For this review, take the finished solid that the model builds, in its own axes (mm). A direction names the side the tool comes from. Coordinates: 2 decimals unless noted, no trailing zeros. Write each loop counter-clockwise with the first axis right and the second up, starting at its lowest first coordinate (ties: lowest second). Pieces come first, ordered by that corner, then holes. Notation, with made-up numbers: (54, 52.5) -> (103, 52.5) arc R16 ccw to (103, 67.5) -> close; hole circle Ø1 at (-19, -2.5). An arc over 180 degrees is marked (long way). Put each result on its own line as item: value. Start each with the question number.
Item 1: Consider section D-D on z = 3. Give the boundary of the cut face in (x, y).
Item 2: Consider section C-C on x = 68.5. Give the boundary of the cut face in (y, z).
Item 3: For faces 4 (the flat face through (137.496, -8.802, 8.208)), 5 (the cylindrical face through (134.365, 3.488, -8.837)), 6 (the flat face through (134.92, 11, -4)), list the 3-axis set-ups (+Z, -Z, +X, -X, +Y, -Y) from which the entire face can be reached by the end or side of a thin tool; tool diameter is ignored.
Item 4: Consider section A-A on y = 0. Give the boundary of the cut face in (x, z).
Item 5: The part is to be moulded in two halves that separate along X. For faces 1 (the flat face through (0, 0, 0)), 2 (the flat face through (137, 12, 0)), 3 (the flat face through (134.92, -11, 4)), say which applies: +X half, -X half, draft (parallel to the pull), parting line (faces both ways), or undercut.
Item 6: To check wall thickness, follow L1, parallel to X at y = -0.5, z = -10; L2, parallel to X at y = 18, z = -11.5; L3, parallel to Y at x = 121.5, z = -14.5. State the ranges of each line that lie inside material, in increasing order.
Item 7: Insertion check: P1, Ø12, axis at x = 123, z = 0.5, coming from the +Y side; P2, Ø4, axis at x = 75.5, z = -7, coming from the -Y side; P3, Ø8, axis at y = 14.5, z = 18, coming from the +X side. Each pin has a flat end and moves straight along its axis. Give the tip position at first contact, or say it passes through.
Item 8: Consider section B-B on z = -3.5. Give the boundary of the cut face in (x, y), and give its area (3 significant figures).
Autodesk Inventor part; units mm, degrees
ref_plane "YZ Plane" through (0, 0, 0) normal (1, 0, 0) x (0, 1, 0)
ref_plane "XZ Plane" through (0, 0, 0) normal (0, 1, 0) x (-1, 0, 0)
ref_plane "XY Plane" through (0, 0, 0) normal (0, 0, 1) x (1, 0, 0)
sketch "Sketch1" plane through (0, 0, 0) normal (1, 0, 0) x (0, 1, 0)
  circle A0 centre (0, 0) radius 15
  dimension "d0" = 30
extrude "Extrusion1" add sketch "Sketch1" along normal blind 140
sketch "Sketch2" plane through (140, 0, 0) normal (1, 0, 0) x (0, 0, -1)
  circle A0 centre (0, 0) radius 9.5
  circle A1 centre (0, 0) radius 15
  line L0 (0, 15) -> (0, 9.5)
  line L1 (0, -9.5) -> (0, -15)
  line L2 (10.23, 10.9703) -> (6.479, 6.9479)
  line L3 (-10.23, -10.9703) -> (-6.479, -6.9479)
  dimension "d3" = 19
  dimension "d4" = 43
  dimension "d5" = 43
extrude "Extrusion2" cut sketch "Sketch2" against normal blind 11.43 contours A0 L2 A1 L1 | A0 L3 A1 L0
sketch "Sketch3" plane through (128.57, 0, 0) normal (1, 0, 0) x (0, 0, -1)
  circle A0 centre (0, 0) radius 15
  circle A1 centre (0, 0) radius 9.5
  dimension "d22" = 19
  dimension "d23" = 30
extrude "Extrusion3" cut sketch "Sketch3" along normal blind 6.35
sketch "Sketch6" plane through (0, 0, 0) normal (-1, 0, 0) x (0, 0, 1)
  circle A0 centre (0, 0) radius 22.5
  dimension "d16" = 45
extrude "Extrusion6" add sketch "Sketch6" against normal up to surface (128.57 mm away)
sketch "Sketch7" plane through (0, 0, 0) normal (-1, 0, 0) x (0, 0, 1)
  circle A0 centre (0, 0) radius 15
  circle A1 centre (0, 0) radius 22.5
  dimension "d19" = 30
extrude "Extrusion7" cut sketch "Sketch7" against normal blind 11.43
sketch "Sketch8" plane through (140, 0, 0) normal (1, 0, 0) x (0, 0, -1)
  arc A0 (10.23, 10.9703) -> (0, 15) centre (0, 0) ccw
  circle A1 centre (0, 0) radius 15
  circle A2 centre (0, 0) radius 14.5
  point P0 (0, 15)
  dimension "d24" = 0.5
extrude "Extrusion8" cut sketch "Sketch8" against normal up to surface (5.08 mm away)
properties part number "spool axle" material "PLA"
Return value:
1. outline: (0, -14.7) -> (11.43, -14.7) -> (11.43, -22.3) -> (128.57, -22.3) -> (128.57, -9.01) -> (134.92, -9.01) -> (134.92, -14.19) -> (140, -14.19) -> (140, 9.01) -> (128.57, 9.01) -> (128.57, 22.3) -> (11.43, 22.3) -> (11.43, 14.7) -> (0, 14.7) -> close
2. outline: circle Ø45 at (0, 0)
3. face 4: +Z, +X
3. face 5: none
3. face 6: -Z, +Y
4. outline: (0, -15) -> (11.43, -15) -> (11.43, -22.5) -> (128.57, -22.5) -> (128.57, -9.5) -> (140, -9.5) -> (140, 9.5) -> (128.57, 9.5) -> (128.57, 22.5) -> (11.43, 22.5) -> (11.43, 15) -> (0, 15) -> close
5. face 1: -X half
5. face 2: draft
5. face 3: undercut
6. L1: 0 to 128.57
6. L2: 11.43 to 128.57
6. L3: -17.2 to 17.2
7. P1: y = 22.5
7. P2: y = -21.94
7. P3: x = 128.57
8. outline: (0, -14.59) -> (11.43, -14.59) -> (11.43, -22.23) -> (128.57, -22.23) -> (128.57, -8.83) -> (140, -8.83) -> (140, 14.07) -> (134.92, 14.07) -> (134.92, 8.83) -> (128.57, 8.83) -> (128.57, 22.23) -> (11.43, 22.23) -> (11.43, 14.59) -> (0, 14.59) -> close
8. area: 5,770 mm^2
